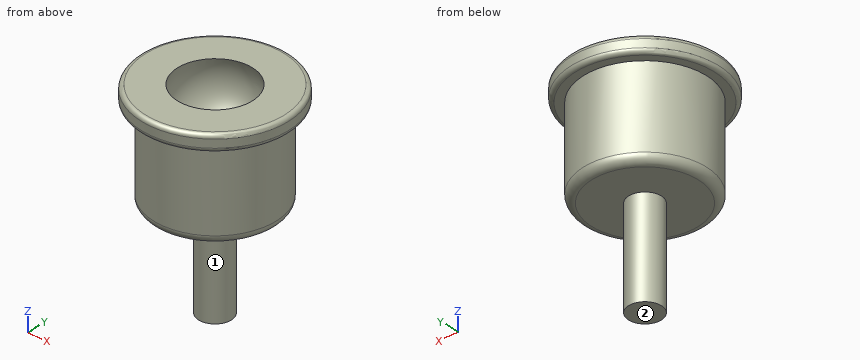
Autodesk Inventor part; units mm, degrees
ref_plane "Work Plane1" through (0, 0, 7.1438) normal (0, 0, 1) x (1, 0, 0)
ref_plane "YZ Plane" through (0, 0, 0) normal (1, 0, 0) x (0, 1, 0)
ref_plane "XZ Plane" through (0, 0, 0) normal (0, 1, 0) x (-1, 0, 0)
sketch "Sketch1" plane through (0, 0, 0) normal (0, 0, 1) x (1, 0, 0)
  circle A0 centre (0, 0) radius 14.2875
  dimension "d0" = 28.575
extrude "Extrusion1" add sketch "Sketch1" along normal mid plane 20.6375
sketch "Sketch2" plane through (0, 0, -10.3188) normal (0, 0, -1) x (-1, 0, 0)
  circle A0 centre (0, 0) radius 14.2875
  circle A1 centre (0, 0) radius 11.9062
  dimension "d3" = 23.8125
extrude "Extrusion2" cut sketch "Sketch2" against normal blind 17.4625
sketch "Sketch3" plane through (0, 0, -10.3188) normal (0, 0, -1) x (-1, 0, 0)
  circle A0 centre (0, 0) radius 11.9062
  circle A1 centre (0, 0) radius 3.175
  dimension "d6" = 6.35
extrude "Extrusion3" add sketch "Sketch3" along normal blind 19.05 contours A1
thread "Thread1"
ref_plane "Work Plane1" through (0, 0, 7.1438) normal (0, 0, 1) x (1, 0, 0)
sketch "Sketch4" plane through (0, 0, 7.1438) normal (0, 0, 1) x (1, 0, 0)
  line L0 (-20.0025, 0) -> (20.0025, 0)
  line L1 (0, -20.0025) -> (0, 20.0025)
  arc A0 (0, -7.9375) -> (0, 7.9375) centre (0, 0) ccw
  line L2 (0, -7.9375) -> (0, 7.9375)
  dimension "d12" = 15.875
revolve "Revolution1" cut sketch "Sketch4" angle 360 about axis through (0, -10, 7.1438) along (0, 1, 0)
fillet "Fillet1" radius 1.5875 1 edges at (11.9062, 0, -10.3188)
fillet "Fillet2" radius 0.7937 1 edges at (-14.2875, 0, 7.1438)
fillet "Fillet3" radius 0.7937 1 edges at (-14.2875, 0, 10.3188)
properties part number "transfer_housing" material "Steel"
For this review, take the finished solid that the model builds, in its own axes (mm). Face numbers are marked on the shaded views. A direction names the side the tool comes from. Round coordinates to 2 decimals unless told otherwise and drop trailing zeros. Order: outer loops, then holes, each group sorted by start corner. A loop starts at its lowest first (then second) coordinate and runs counter-clockwise, first axis right, second up. Notation, with made-up numbers: (24.5, -14.5) -> (47.5, -14.5) arc R24 ccw to (47.5, 2.5) -> close; hole circle Ø6 at (-25.5, -28.75). An arc over 180 degrees is marked (long way). Put each result on its own line as item: value.
Q1. Add section D-D on z = -26. Write out the cut boundary in (x, y) (3 decimals), plus the area to 3 significant figures.
Check result:
outline: circle Ø6.35 at (0, 0)
area: 31.7 mm2
Q2. Machinability: for the marked faces 1 and 2, which of the approach directions +Z, -Z, +X, -X, +Y, -Y give a long, thin tool a straight path to every point of the face, cutting with its end or side? Answer none if there is none.
Check result:
face 1: -Z
face 2: -Z, +X, -X, +Y, -Y
Q3. Insertion check: pin 1 Ø2 at (y, z) = (-5.5, 0) entering from +X; pin 2 Ø6 at (x, y) = (1, -11) entering from -Z; pin 3 Ø6 at (x, z) = (4.5, -14) entering from -Y; pin 4 Ø16.5 at (x, y) = (-4.5, -5) entering from -Z. Each pin has a flat end and moves straight along its axis. Give the tip position at first contact, or say it passes through.
Check result:
pin 1: x = 11.02
pin 2: z = -10.32
pin 3: y = -2.8
pin 4: z = -29.37
Q4. For probe 1 along Y at (x, z) = (3.25, 3.5); probe 2 along Z at (x, y) = (10, -6.75); probe 3 along Z at (x, y) = (-8, -4), list the stretches that pass through material, from the lowest coordinate up. Write a range as [from, to].
Check result:
probe 1: [-11.45, -6.26], [6.26, 11.45]
probe 2: [7.14, 10.32]
probe 3: [-10.32, 10.32]
Q5. Add section A-A on x = 0. Write out the cut boundary in (y, z) (1 decimal).
Check result:
outline: (-14.3, 7.9) arc R0.8 ccw to (-13.5, 7.1) -> (-11.9, 7.1) -> (-11.9, -8.7) arc R1.6 ccw to (-10.3, -10.3) -> (-3.2, -10.3) -> (-3.2, -29.4) -> (3.2, -29.4) -> (3.2, -10.3) -> (10.3, -10.3) arc R1.6 ccw to (11.9, -8.7) -> (11.9, 7.1) -> (13.5, 7.1) arc R0.8 ccw to (14.3, 7.9) -> (14.3, 9.5) arc R0.8 ccw to (13.5, 10.3) -> (7.3, 10.3) arc R7.9 cw (long way) to (-7.3, 10.3) -> (-13.5, 10.3) arc R0.8 ccw to (-14.3, 9.5) -> close
Q6. Add section C-C on z = -2. Write out the cut boundary in (x, y), plus the area to 3 significant figures.
Check result:
outline: circle Ø23.81 at (0, 0)
area: 445 mm2
